Input: part model. Units: mm. Frame: model coordinates. Round coordinates to 2 decimals unless told otherwise and drop trailing zeros. Order: outer loops, then holes, each group sorted by start corner. A loop starts at its lowest first (then second) coordinate and runs counter-clockwise, first axis right, second up. Notation, with made-up numbers: (87.5, 77.5) - (118.5, 77.5) arc R13 ccw to (118.5, 96.5) - close; hole circle Ø7 at (24.25, -8.5). An arc over 180 degrees is marked (long way). One line per item, written item: value. Start each with the question number.
from build123d import *

# Parameters (mm, degrees)
F0_R     = 2.5527
F1_DEPTH = 3.175


with BuildPart() as f1:
    # F0 (on Front) → F1 (new body)
    with BuildSketch(Plane.XZ):
        Polygon((0, 288.925), (0, 0), (342.9, 0), (342.9, 288.925), (241.3, 288.925), (241.3, 152.4), (101.6, 152.4), (101.6, 288.925), align=None)
        with Locations((181.0013651848, 25.4)):
            Circle(F0_R, mode=Mode.SUBTRACT)
        with Locations((206.4013651848, 25.4)):
            Circle(F0_R, mode=Mode.SUBTRACT)
        with Locations((330.2, 22.225)):
            Circle(F0_R, mode=Mode.SUBTRACT)
        with Locations((330.2, 47.625)):
            Circle(F0_R, mode=Mode.SUBTRACT)
        with Locations((330.2, 73.025)):
            Circle(F0_R, mode=Mode.SUBTRACT)
        with Locations((330.2, 98.425)):
            Circle(F0_R, mode=Mode.SUBTRACT)
        with Locations((330.2, 123.825)):
            Circle(F0_R, mode=Mode.SUBTRACT)
        with Locations((330.2, 149.225)):
            Circle(F0_R, mode=Mode.SUBTRACT)
        with Locations((330.2, 174.625)):
            Circle(F0_R, mode=Mode.SUBTRACT)
        with Locations((330.2, 200.025)):
            Circle(F0_R, mode=Mode.SUBTRACT)
        with Locations((330.2, 225.425)):
            Circle(F0_R, mode=Mode.SUBTRACT)
        with Locations((330.2, 250.825)):
            Circle(F0_R, mode=Mode.SUBTRACT)
    extrude(amount=F1_DEPTH)


solid = f1.part
Item 1: Line query: L1, parallel to X at y = -1.2, z = 230.5; L2, parallel to X at y = -1.1, z = 47.5; L3, parallel to Z at x = 165, y = -2.95. Output: solid intervals per line, ascending.
Item 2: Section query C-C on x = 187.5. Return loops of the section in (y, z) (3 decimals).
Item 3: First-contact query: pin 1 Ø1 at (x, y) = (188, -2) entering from +Z. Flat tip, straight axial feed; report the tip coordinate or a pass-through.
Item 4: Section query B-B on y = -0.6. Give the number of separate pieces and of enclosed holes in the cut face, and give its area (3 significant figures).
Item 5: Section query A-A on z = 184. Return loops of the section in (x, y) (3 decimals).
Geometry results:
1. L1: x = 0 to 101.6, 241.3 to 342.9
1. L2: x = 0 to 327.65, 332.75 to 342.9
1. L3: z = 0 to 152.4
2. outline: (-3.175, 0) - (0, 0) - (0, 152.4) - (-3.175, 152.4) - close
3. pin 1: stops at z = 152.4
4. separate pieces: 1
4. enclosed holes: 12
4. area: 79,800 mm^2
5. outline: (0, -3.175) - (101.6, -3.175) - (101.6, 0) - (0, 0) - close; (241.3, -3.175) - (342.9, -3.175) - (342.9, 0) - (241.3, 0) - close
